Part model, mm, in its own coordinate system. A direction names the side the tool comes from. Round coordinates to 2 decimals unless told otherwise and drop trailing zeros. Loops run counter-clockwise (first coordinate to the right, second up) from the corner with the lowest first, then second, coordinate; pieces in that order, holes last. Notation, with made-up numbers: (-14.5, -32.5) -> (-1.5, -32.5) arc R18 cw to (-1.5, 0.5) -> close; hole circle Ø4 at (88.5, 58.5). An arc over 180 degrees is marked (long way). Answer as CSV lines item,"result".
from build123d import *

# Parameters (mm, degrees)
SKETCH2_R           = 5.25
BOSS_EXTRUDE1_DEPTH = 12.3
CHAMFER1_SIZE       = 1.5
CHAMFER2_SIZE       = 12
FILLET1_R           = 1


with BuildPart() as part:
    # Sketch2 → Boss-Extrude1 (new body)
    with BuildSketch(Plane(origin=(0, 0, 0), x_dir=(1, 0, 0), z_dir=(0, 1, 0))):
        Polygon((-50, 10), (-50, -10), (-15, -10), (-6.5, -10), (-6.5, 10), align=None)
        with Locations((-30.066740906, -2)):
            Circle(SKETCH2_R, mode=Mode.SUBTRACT)
        Polygon((-6.5, -10), (-15, -10), (-15, -31.53738907), (15, -31.53738907), (15, -10), (6.5, -10), (6.5, -21.6), (-6.5, -21.6), align=None)
        Polygon((6.5, 10), (6.5, -10), (15, -10), (50, -10), (50, 10), align=None)
        with Locations((29.933259094, -2)):
            Circle(SKETCH2_R, mode=Mode.SUBTRACT)
    extrude(amount=BOSS_EXTRUDE1_DEPTH)

    # Chamfer1
    chamfer1_edges = [part.edges().sort_by_distance(p)[0] for p in [
        (-35.316740906, 12.3, 2),
        (24.683259094, 12.3, 2),
    ]]
    chamfer(chamfer1_edges, length=CHAMFER1_SIZE)

    # Chamfer2
    chamfer2_edges = [part.edges().sort_by_distance(p)[0] for p in [
        (6.5, 6.15, -10),
        (-6.5, 6.15, -10),
    ]]
    chamfer(chamfer2_edges, length=CHAMFER2_SIZE)

    # Fillet1
    fillet1_edges = [part.edges().sort_by_distance(p)[0] for p in [
        (50, 0, 0),
        (32.5, 0, 10),
        (15, 0, 20.768694535),
        (0, 0, 31.53738907),
        (-15, 0, 20.768694535),
        (-32.5, 0, 10),
        (-50, 0, 0),
        (-34.25, 0, -10),
        (-18.5, 6.15, -10),
        (-6.5, 0, 11.8),
        (6.5, 0, 11.8),
        (34.25, 0, -10),
        (12.5, 0, -4),
        (-12.5, 0, -4),
        (-6.5, 6.15, 2),
        (6.5, 6.15, 2),
        (18.5, 6.15, -10),
    ]]
    fillet(fillet1_edges, radius=FILLET1_R)


solid = part.part
Q1. Two-plate mould, pull along X, no slides. Class faces 1 (the face through (50, 7, 0)), 2 (the face through (-50, 7, 0)), 3 (the face through (35, 11, 0)): pulls with the +X half, pulls with the -X half, needs draft (parallel to the pull), parting line crosses it, or undercut.
Geometry results:
face 1,"pulls with the +X half"
face 2,"pulls with the -X half"
face 3,"undercut"
Q2. Drop flat-ended pins along their axis: P1, Ø8, axis at x = 7, z = 7, coming from the -Y side; P2, Ø5.5, axis at y = 6, z = 22.5, coming from the +X side; P3, Ø5, axis at x = 29, y = 6.5, coming from the +Z side; P4, Ø3, axis at y = 2, z = 21, coming from the -X side. Give the stop position or say it passes through.
Geometry results:
P1,"y = 0"
P2,"x = 15"
P3,"z = 10"
P4,"x = -15"
Q3. Drill centre lines: line 1 along X through (y, z) = (8.75, 17); line 2 along X through (y, z) = (10.5, -1.5); line 3 along X through (y, z) = (7, 2). Where is each one in solid material? Low to high.
Geometry results:
line 1,"-15 to -6.5, 6.5 to 15"
line 2,"-50 to -33.98, -26.15 to -10, 10 to 26.02, 33.85 to 50"
line 3,"-50 to -35.32, -24.82 to -6.59, 6.59 to 24.68, 35.18 to 50"
Q4. Saw through at A-A, the plane z = 18.5. Write the cut outline in (x, y).
Geometry results:
outline,"(-15, 1) arc R1 ccw to (-14, 0) -> (-7.5, 0) arc R1 ccw to (-6.5, 1) -> (-6.5, 12.3) -> (-15, 12.3) -> close; (6.5, 1) arc R1 ccw to (7.5, 0) -> (14, 0) arc R1 ccw to (15, 1) -> (15, 12.3) -> (6.5, 12.3) -> close"
Q5. Saw through at D-D, the plane x = 21. Write the cut outline in (y, z), then the cut area to 3 significant figures.
Geometry results:
outline,"(0, -9) arc R1 ccw to (1, -10) -> (12.3, -10) -> (12.3, 10) -> (1, 10) arc R1 ccw to (0, 9) -> close"
area,"246 mm2"
Q6. Saw through at C-C, the plane x = 5. Write the cut outline in (y, z).
Geometry results:
outline,"(0, 21.6) -> (12.3, 21.6) -> (12.3, 31.54) -> (1, 31.54) arc R1 ccw to (0, 30.54) -> close"
Q7. Saw through at B-B, the plane y = 5. Write the cut outline in (x, z), then the cut area to 3 significant figures.
Geometry results:
outline,"(-50, -10) -> (-18.91, -10) arc R1 ccw to (-18.21, -9.71) -> (-6.79, 1.71) arc R1 ccw to (-6.5, 2.41) -> (-6.5, 21.6) -> (6.5, 21.6) -> (6.5, 2.41) arc R1 ccw to (6.79, 1.71) -> (18.21, -9.71) arc R1 ccw to (18.91, -10) -> (50, -10) -> (50, 10) -> (15, 10) -> (15, 31.54) -> (-15, 31.54) -> (-15, 10) -> (-50, 10) -> close; hole circle Ø10.5 at (-30.07, 2); hole circle Ø10.5 at (29.93, 2)"
area,"1,920 mm2"
Q8. Which spindle directions (+Z, -Z, +X, -X, +Y, -Y) get a long thin tool onto all of the face, cutting with end or side? Do faces 4 (the face through (6.5, 7, 12)), 5 (the face through (-15, 7, 21)), 6 (the face through (32, 7, 10)), 7 (the face through (-12.63, 0.29, -3.71)). Say none if no direction does.
Geometry results:
face 4,"-Z, +Y, -Y"
face 5,"+Z, -X, +Y, -Y"
face 6,"+Z, +X, +Y, -Y"
face 7,"-Z, -Y"
